from build123d import *

# Parameters (mm, degrees)
F0_W     = 76.2
F0_H     = 76.2
F1_DEPTH = 10
F3_DEPTH = 7
F5_DEPTH = 7.25
F6_W     = 19.3
F6_H     = 3.25
F8_DEPTH = 6.6
F9_COUNT = 4
F9_ANGLE = 270
F11_SIZE = 0.5


with BuildPart() as f1:
    # F0 (on Top) → F1 (new body)
    with BuildSketch(Plane.XY):
        Rectangle(F0_W, F0_H)
    extrude(amount=F1_DEPTH)

    # F2 (on face) → F3 (join)
    with BuildSketch(Plane.XY.offset(10)):
        Polygon((5, -2.8867513459), (5, 2.8867513459), (0, 5.7735026919), (-5, 2.8867513459), (-5, -2.8867513459), (0, -5.7735026919), align=None)
    extrude(amount=F3_DEPTH)

    # F4 (on face) → F5 (cut)
    with BuildSketch(Plane(origin=(0, 0, 0), x_dir=(1, 0, 0), z_dir=(0, 0, -1))):
        Polygon((5.25, -3.0310889132), (5.25, 3.0310889132), (0, 6.0621778265), (-5.25, 3.0310889132), (-5.25, -3.0310889132), (0, -6.0621778265), align=None)
    extrude(amount=-F5_DEPTH, mode=Mode.SUBTRACT)


with BuildPart() as f8:
    # F6 (on face) → F8 (new body)
    with BuildSketch(Plane.XZ.offset(38.1)):
        with Locations((-19.05, 5)):
            Rectangle(F6_W, F6_H)
    extrude(amount=-F8_DEPTH)


with BuildPart() as f8b:
    # F6 (on face) → F8, piece 2 (new body)
    with BuildSketch(Plane.XZ.offset(38.1)):
        with Locations((19.05, 5)):
            Rectangle(F6_W, F6_H)
    extrude(amount=-F8_DEPTH)


with BuildPart() as f9_1:
    # F9: instance of F8b
    add(f8b.part.rotate(Axis((0, 0, 20.068032667), (0, 0, -1)), 1 * F9_ANGLE / (F9_COUNT - 1)))


with BuildPart() as f9_2:
    # F9: instance of F8b
    add(f8b.part.rotate(Axis((0, 0, 20.068032667), (0, 0, -1)), 2 * F9_ANGLE / (F9_COUNT - 1)))


with BuildPart() as f9_3:
    # F9: instance of F8b
    add(f8b.part.rotate(Axis((0, 0, 20.068032667), (0, 0, -1)), 3 * F9_ANGLE / (F9_COUNT - 1)))


with BuildPart() as f9_4:
    # F9: instance of F8
    add(f8.part.rotate(Axis((0, 0, 20.068032667), (0, 0, -1)), 1 * F9_ANGLE / (F9_COUNT - 1)))


with BuildPart() as f9_5:
    # F9: instance of F8
    add(f8.part.rotate(Axis((0, 0, 20.068032667), (0, 0, -1)), 2 * F9_ANGLE / (F9_COUNT - 1)))


with BuildPart() as f9_6:
    # F9: instance of F8
    add(f8.part.rotate(Axis((0, 0, 20.068032667), (0, 0, -1)), 3 * F9_ANGLE / (F9_COUNT - 1)))


with BuildPart() as f1_1:
    add(f1.part)

    # F10: cut F9_3, F9_6, F9_2, F9_5, F9_1, F9_4, F8b, F8
    add(f9_3.part, mode=Mode.SUBTRACT)
    add(f9_6.part, mode=Mode.SUBTRACT)
    add(f9_2.part, mode=Mode.SUBTRACT)
    add(f9_5.part, mode=Mode.SUBTRACT)
    add(f9_1.part, mode=Mode.SUBTRACT)
    add(f9_4.part, mode=Mode.SUBTRACT)
    add(f8b.part, mode=Mode.SUBTRACT)
    add(f8.part, mode=Mode.SUBTRACT)

    # F11
    f11_edges = [f1_1.edges().sort_by_distance(p)[0] for p in [
        (5, 0, 17),
        (2.5, 4.330127, 17),
        (-2.5, 4.330127, 17),
        (-5, 0, 17),
        (-2.5, -4.330127, 17),
        (2.5, -4.330127, 17),
        (2.625, 4.546633, 0),
        (5.25, 0, 0),
        (2.625, -4.546633, 0),
        (-2.625, -4.546633, 0),
        (-5.25, 0, 0),
        (-2.625, 4.546633, 0),
        (38.1, -19.05, 6.625),
        (38.1, -9.4, 5),
        (38.1, -19.05, 3.375),
        (38.1, -28.7, 5),
        (38.1, 19.05, 3.375),
        (38.1, 9.4, 5),
        (38.1, 28.7, 5),
        (38.1, 19.05, 6.625),
        (19.05, 38.1, 6.625),
        (28.7, 38.1, 5),
        (9.4, 38.1, 5),
        (19.05, 38.1, 3.375),
        (28.7, -38.1, 5),
        (19.05, -38.1, 6.625),
        (9.4, -38.1, 5),
        (19.05, -38.1, 3.375),
        (-9.4, -38.1, 5),
        (-19.05, -38.1, 6.625),
        (-19.05, -38.1, 3.375),
        (-28.7, -38.1, 5),
        (-38.1, -28.7, 5),
        (-38.1, -19.05, 6.625),
        (-38.1, -9.4, 5),
        (-38.1, -19.05, 3.375),
        (-38.1, 9.4, 5),
        (-38.1, 19.05, 6.625),
        (-38.1, 28.7, 5),
        (-38.1, 19.05, 3.375),
        (-19.05, 38.1, 6.625),
        (-28.7, 38.1, 5),
        (-9.4, 38.1, 5),
        (-19.05, 38.1, 3.375),
    ]]
    chamfer(f11_edges, length=F11_SIZE)


solid = f1_1.part
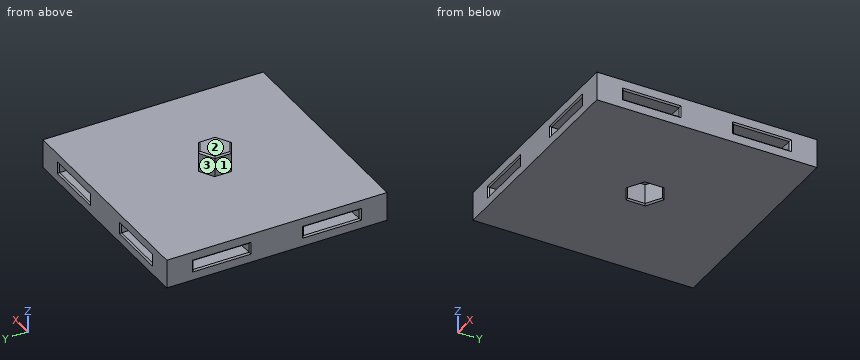
For this review, take the finished solid that the model builds, in its own axes (mm). Face numbers are marked on the shaded views. A direction names the side the tool comes from. Round coordinates to 2 decimals unless told otherwise and drop trailing zeros. Loops run counter-clockwise (first coordinate to the right, second up) from the corner with the lowest first, then second, coordinate; pieces in that order, holes last. Notation, with made-up numbers: (-34.5, 2) - (11.5, 2) arc R14 cw to (11.5, 12) - close; hole circle Ø8 at (19.5, 22). An arc over 180 degrees is marked (long way). Put each result on its own line as item: value. Start each with the question number.
1. Consider section B-B on y = -27. State the section outline as (x, z) points (3 decimals), plus the area to 3 significant figures.
2. For probe 1 along Y at (x, z) = (32, 4.75); probe 2 along Z at (x, y) = (13, -33) (3 decimals); probe 3 along Z at (x, y) = (27.5, -3), list the stretches that pass through material, from the lowest coordinate up. Write a range as [from, to].
3. For the marked faces 1, 2 and 3, list the 3-axis set-ups (+Z, -Z, +X, -X, +Y, -Y) from which the entire face can be reached by the end or side of a thin tool; tool diameter is ignored.
4. Insertion check: P1, Ø2, axis at x = 16.5, y = -14, coming from the +Z side; P2, Ø3, axis at x = -1.5, y = -2, coming from the -Z side. Each pin has a flat end and moves straight along its axis. Give the tip position at first contact, or say it passes through.
5. Consider section D-D on z = 15.5. State the section outline as (x, y) points, plus the area to 3 significant figures.
6. Consider section A-A on x = -33. State the section outline as (y, z) points (3 decimals).
Result sheet:
1. outline: (-38.1, 0) - (38.1, 0) - (38.1, 2.875) - (37.6, 3.375) - (31.5, 3.375) - (31.5, 6.625) - (37.6, 6.625) - (38.1, 7.125) - (38.1, 10) - (-38.1, 10) - (-38.1, 7.125) - (-37.6, 6.625) - (-31.5, 6.625) - (-31.5, 3.375) - (-37.6, 3.375) - (-38.1, 2.875) - close
1. area: 719 mm^2
2. probe 1: [-38.1, -28.7], [-9.4, 9.4], [28.7, 38.1]
2. probe 2: [0, 3.375], [6.625, 10]
2. probe 3: [0, 10]
3. face 1: +Z, -X, +Y, -Y
3. face 2: +Z, +X, -X, +Y, -Y
3. face 3: +Z, -X, +Y
4. P1: z = 10
4. P2: z = 7.25
5. outline: (-5, -2.89) - (0, -5.77) - (5, -2.89) - (5, 2.89) - (0, 5.77) - (-5, 2.89) - close
5. area: 86.6 mm^2
6. outline: (-38.1, 0) - (38.1, 0) - (38.1, 10) - (-38.1, 10) - close; hole (-28.7, 3.375) - (-9.4, 3.375) - (-9.4, 6.625) - (-28.7, 6.625) - close; hole (9.4, 3.375) - (28.7, 3.375) - (28.7, 6.625) - (9.4, 6.625) - close
